Answer from the drawing. Dimensions are ordinates in mm from the lowest x, y and z of the part. Coordinates: 2 decimals unless noted, no trailing zeros. Write each loop counter-clockwise with the first axis right and the second up, starting at its lowest first coordinate (ties: lowest second). Pieces come first, ordered by that corner, then holes.
(1) The part is cut by section D-D on y = 54. Determine the outline of the cut face in (x, z), plus the area to 3 significant figures.
(2) The part is cut by section C-C on z = 1.3. Determine the outline of the cut face in (x, y), plus the area to 3 significant figures.
(3) Given P1, Ø3, axis at x = 70, y = 36.5, coming from the -Z side, flat-ended and moving along its own axis, determine where the tip first touches the part or whether it passes through.
(4) The part is cut by section A-A on x = 40. Determine the outline of the cut face in (y, z), plus the area to 3 significant figures.
(5) Straight lines are drawn through the part: line 1 (Y direction, x = 35.5, z = 0.15); line 2 (X direction, y = 76, z = 0.8); line 3 (Y direction, x = 105, z = 1.8). For each, find the intervals that lie inside material, in ascending order.
(6) The part is cut by section B-B on y = 81. Determine the outline of the cut face in (x, z).
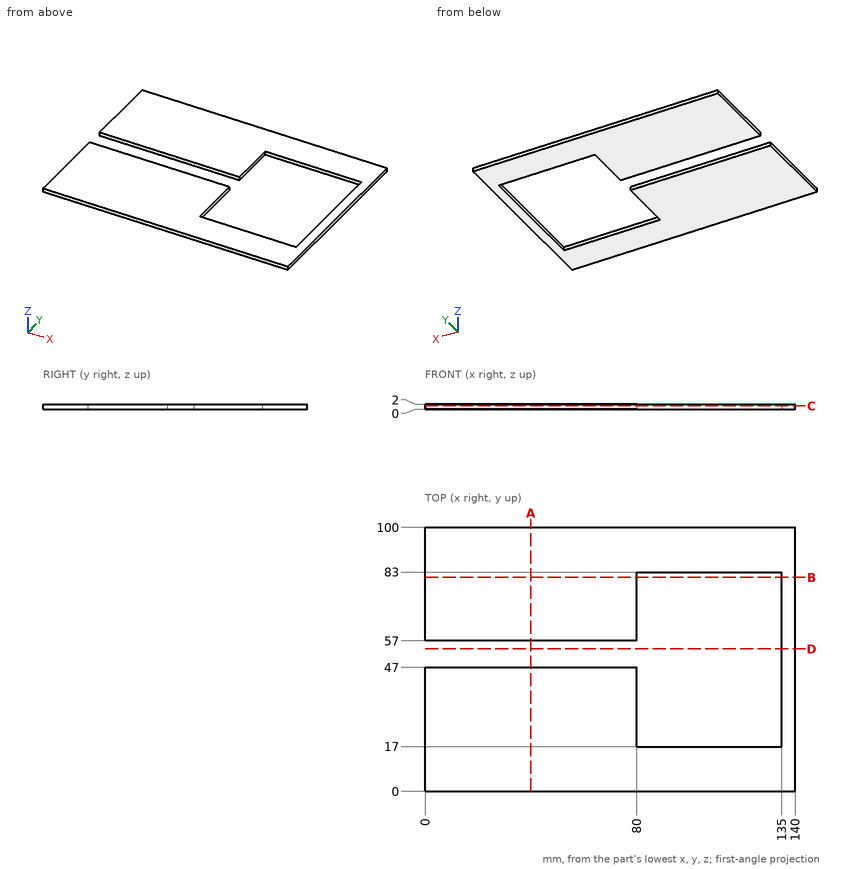
Model answer:
1. outline: (135, 0) - (140, 0) - (140, 2) - (135, 2) - close
1. area: 10.0 mm2
2. outline: (0, 0) - (140, 0) - (140, 100) - (0, 100) - (0, 57) - (80, 57) - (80, 83) - (135, 83) - (135, 17) - (80, 17) - (80, 47) - (0, 47) - close
2. area: 9,570 mm2
3. P1: stops at z = 0
4. outline: (0, 0) - (47, 0) - (47, 2) - (0, 2) - close; (57, 0) - (100, 0) - (100, 2) - (57, 2) - close
4. area: 180 mm2
5. line 1: y = 0 to 47, 57 to 100
5. line 2: x = 0 to 80, 135 to 140
5. line 3: y = 0 to 17, 83 to 100
6. outline: (0, 0) - (80, 0) - (80, 2) - (0, 2) - close; (135, 0) - (140, 0) - (140, 2) - (135, 2) - close
